Source: CAD feature listing. Evaluate the final solid. Frame: model axes, mm. Face numbers are marked on the shaded views. A direction names the side the tool comes from. Round coordinates to 2 decimals unless told otherwise and drop trailing zeros. Loops run counter-clockwise (first coordinate to the right, second up) from the corner with the lowest first, then second, coordinate; pieces in that order, holes last. Notation, with made-up numbers: M -23,42.5 L -3,42.5 A12 cw -3,51.5 Z; hole C 28.5,-9 d11. An arc over 180 degrees is marked long. Write each question's results on one line, items separated by ' | '. Start each with the question number.
1. Section C-C on z = 3.75. Output: boundary loops of the cut face in (x, y).
2. Contact query for flat-ended pins moving along their axis: pin 1 Ø2 at (x, z) = (-21.5, 13) entering from +Y; pin 2 Ø5 at (y, z) = (-10, 9) entering from -X; pin 3 Ø5 at (y, z) = (20.5, 12) entering from +X. Output: stop coordinate, or through.
3. Section A-A on y = 0. Output: boundary loops of the cut face in (x, z).
4. Set-up query: the marked faces 1, 2 and 3. Return all of +Z, -Z, +X, -X, +Y, -Y with unobstructed straight access to the full face (end or side cutting, diameter ignored); none if empty.
5. Section B-B on x = 0. Output: boundary loops of the cut face in (y, z).
6. Draft query along X for the marked faces 4, 5 and 6. Return one class per face: released by +X, released by -X, zero draft, split by the parting line, or undercut.
7. Section D-D on z = 15.25. Output: boundary loops of the cut face in (x, y), and give its area (3 significant figures).
8. Ray query, line 1 (Y direction, x = 0, z = 10.5); line 2 (X direction, y = -1.5, z = 12.75); line 3 (Y direction, x = 15.5, z = 13). Return the intervals inside material, ascending.
Autodesk Inventor part; units mm, degrees
ref_plane "Arbeitsebene1" through (0, 0, 3) normal (0, 0, -1) x (-1, 0, 0)
ref_plane "Arbeitsebene2" through (0, 0, 7) normal (0, 0, -1) x (-1, 0, 0)
ref_plane "YZ Plane" through (0, 0, 0) normal (1, 0, 0) x (0, 1, 0)
sketch "Skizze2" plane through (0, 0, 0) normal (0, 0, 1) x (1, 0, 0)
  circle A0 centre (0, 0) radius 30
  dimension "d0" = 60
extrude "Extrusion1" add sketch "Skizze2" along normal blind 17
sketch "Skizze8" plane through (0, 0, 17) normal (0, 0, 1) x (1, 0, 0)
  circle A0 centre (0, 0) radius 30
hole "Bohrung1" at (0, 0, 17) direction (0, 0, -1) diameter 47.5 end through all
ref_plane "Arbeitsebene1" through (0, 0, 3) normal (0, 0, -1) x (-1, 0, 0)
ref_plane "Arbeitsebene2" through (0, 0, 7) normal (0, 0, -1) x (-1, 0, 0)
sketch "Skizze6" plane through (0, 0, 17) normal (0, 0, 1) x (1, 0, 0)
  circle A0 centre (0, 0) radius 23.75
  circle A1 centre (0, 0) radius 30
  circle A2 centre (0, 0) radius 27.5
  dimension "d34" = 55
extrude "Extrusion4" cut sketch "Skizze6" against normal up to surface (4 mm away) from surface at -10 contours A2
sketch "Skizze7" plane through (0, 0, 17) normal (0, 0, 1) x (1, 0, 0)
  circle A0 centre (0, 0) radius 30
hole "Bohrung2" at (0, 0, 17) direction (0, 0, -1) diameter 53.5 depth 10 tip angle 118
thread "Gewinde3"
chamfer "Fase4" distance 1 angle 45 1 edges at (-30, 0, 0)
sketch "Skizze9" plane through (0, 0, 0) normal (0, 0, -1) x (-1, 0, 0)
  point P0 (0, 0)
  point P1 (23.75, 0)
  dimension "d51" = 23.75
hole "Bohrung3" at (-23.75, 0, 0) direction (0, 0, 1) diameter 6 end through all
equation "\"Biegeradius\" = Stärke"
equation "\"BreiteBiegungsfreistellung\" = Stärke"
equation "\"TiefeBiegungsfreistellung\" = 0.5 * Stärke"
equation "\"GrößeEckenfreistellung\" = 4 * Stärke"
equation "\"MinimalRest\" = 2 * Stärke"
equation "\"Übergangsradius\" = Biegeradius"
equation "\"JacobiRadiusGröße\" = Stärke"
equation "\"Abstandsgröße\" = Stärke"
properties part number "Überwurfmutter" material "PC/ABS-Kunststoff"
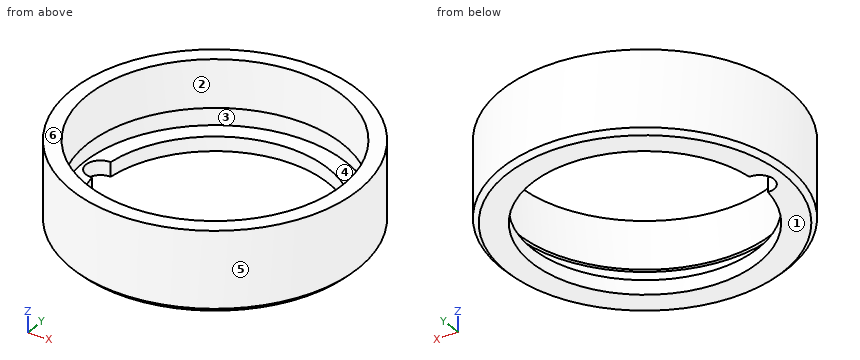
Taken from the geometry:
1) outline: C 0,0 d60; hole C 0,0 d55
2) pin 1: y = 21.9 | pin 2: x = -29.05 | pin 3: x = 24
3) outline: M -30,1 L -29,0 L -26.75,0 L -26.75,3 L -27.5,3 L -27.5,7 L -26.75,7 L -26.75,17 L -30,17 Z; M 23.75,0 L 29,0 L 30,1 L 30,17 L 26.75,17 L 26.75,7 L 27.5,7 L 27.5,3 L 23.75,3 Z
4) face 1: -Z, +X, -X, +Y, -Y | face 2: +Z | face 3: none
5) outline: M -30,1 L -29,0 L -23.75,0 L -23.75,3 L -27.5,3 L -27.5,7 L -26.75,7 L -26.75,17 L -30,17 Z; M 23.75,0 L 29,0 L 30,1 L 30,17 L 26.75,17 L 26.75,7 L 27.5,7 L 27.5,3 L 23.75,3 Z
6) face 4: undercut | face 5: split by the parting line | face 6: zero draft
7) outline: C 0,0 d60; hole C 0,0 d53.5 | area: 579 mm^2
8) line 1: -30 to -26.75, 26.75 to 30 | line 2: -29.96 to -26.71, 26.71 to 29.96 | line 3: -25.69 to -21.8, 21.8 to 25.69
